Work out the finished part from the listing and answer in its coordinate system (mm). Face numbers are marked on the shaded views. A direction names the side the tool comes from. Coordinates: 2 decimals unless noted, no trailing zeros. Order: outer loops, then holes, each group sorted by start corner. A loop starts at its lowest first (then second) coordinate and runs counter-clockwise, first axis right, second up.
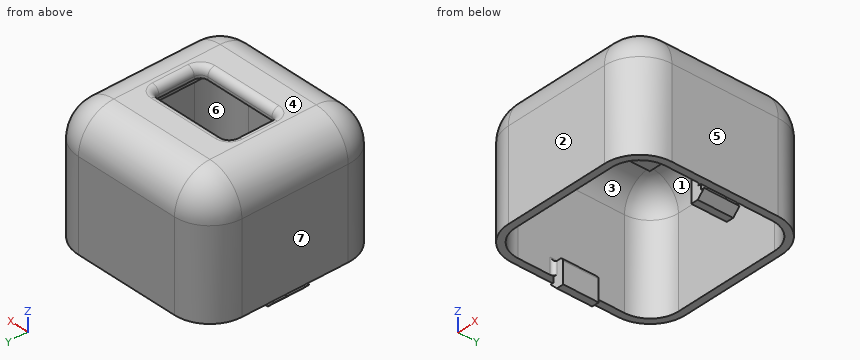
```python
from build123d import *

# Parameters (mm, degrees)
SKETCH1_W                = 50
SKETCH1_H                = 50
BOSS_EXTRUDE1_DEPTH      = 45
FILLET1_R                = 10
SHELL1_T                 = -2
SKETCH2_W                = 24
SKETCH2_H                = 14
CUT_EXTRUDE1_DEPTH       = 10
SKETCH3_W                = 28
SKETCH3_H                = 18
BOSS_EXTRUDE2_DEPTH      = 2
SKETCH4_W                = 24
SKETCH4_H                = 14
CUT_EXTRUDE2_DEPTH       = 2
FILLET2_R                = 2
FILLET3_R                = 2
SKETCH5_W                = 28
SKETCH5_H                = 28
BOSS_EXTRUDE3_DEPTH      = 2
CUT_EXTRUDE4_DEPTH       = 2
SKETCH8_W                = 25
SKETCH8_H                = 17
CUT_EXTRUDE5_DEPTH       = 1.2
SKETCH9_W                = 28
SKETCH9_H                = 4
CUT_EXTRUDE6_DEPTH       = 1.2
CUT_EXTRUDE10_START      = -10
CUT_EXTRUDE10_DEPTH      = 10
SKETCH14_W               = 7
SKETCH14_H               = 10
BOSS_EXTRUDE4_DEPTH      = 3
SKETCH15_W               = 2
SKETCH15_H               = 10
BOSS_EXTRUDE5_DEPTH      = 1
CHAMFER1_SIZE            = 2
FILLET4_R                = 1
CHAMFER1_OF_MIRROR1_SIZE = 2
FILLET5_R                = 1


with BuildPart() as part:
    # Sketch1 → Boss-Extrude1 (new body)
    with BuildSketch(Plane.XY):
        Rectangle(SKETCH1_W, SKETCH1_H)
    extrude(amount=BOSS_EXTRUDE1_DEPTH)

    # Fillet1
    fillet1_edges = [part.edges().sort_by_distance(p)[0] for p in [
        (-25, 0, 45),
        (0, -25, 45),
        (25, 0, 45),
        (25, -25, 22.5),
        (-25, -25, 22.5),
        (-25, 25, 22.5),
        (25, 25, 22.5),
        (0, 25, 45),
    ]]
    fillet(fillet1_edges, radius=FILLET1_R)

    # Shell1
    shell1_openings = [part.faces().sort_by_distance(p)[0] for p in [
        (0, 0, 0),
    ]]
    offset(amount=SHELL1_T, openings=shell1_openings, kind=Kind.INTERSECTION)

    # Sketch2 → Cut-Extrude1 (cut)
    with BuildSketch(Plane(origin=(0, 0, 43), x_dir=(-1, 0, 0), z_dir=(0, 0, -1))):
        Rectangle(SKETCH2_W, SKETCH2_H)
    extrude(amount=-CUT_EXTRUDE1_DEPTH, mode=Mode.SUBTRACT)

    # Sketch3 → Boss-Extrude2 (add)
    with BuildSketch(Plane(origin=(0, 0, 43), x_dir=(-1, 0, 0), z_dir=(0, 0, -1))):
        Rectangle(SKETCH3_W, SKETCH3_H)
    extrude(amount=BOSS_EXTRUDE2_DEPTH)

    # Sketch4 → Cut-Extrude2 (cut)
    with BuildSketch(Plane.XY.offset(43)):
        Rectangle(SKETCH4_W, SKETCH4_H)
    extrude(amount=-CUT_EXTRUDE2_DEPTH, mode=Mode.SUBTRACT)

    # Fillet2
    fillet2_edges = [part.edges().sort_by_distance(p)[0] for p in [
        (-12, 7, 43),
        (-12, -7, 43),
        (12, -7, 43),
        (12, 7, 43),
    ]]
    fillet(fillet2_edges, radius=FILLET2_R)

    # Fillet3
    fillet3_edges = [part.edges().sort_by_distance(p)[0] for p in [
        (12, 0, 45),
        (0, 7, 45),
        (0, -7, 45),
        (-12, 0, 45),
        (11.414213562, 6.414213562, 45),
        (11.414213562, -6.414213562, 45),
        (-11.414213562, -6.414213562, 45),
        (-11.414213562, 6.414213562, 45),
    ]]
    fillet(fillet3_edges, radius=FILLET3_R)

    # Sketch5 → Boss-Extrude3 (add)
    with BuildSketch(Plane(origin=(0, 0, 41), x_dir=(-1, 0, 0), z_dir=(0, 0, -1))):
        Rectangle(SKETCH5_W, SKETCH5_H)
    extrude(amount=-BOSS_EXTRUDE3_DEPTH)

    # Sketch7 → Cut-Extrude4 (cut)
    with BuildSketch(Plane.XY.offset(43)):
        with BuildLine():
            Line((12, -5), (12, 5))
            ThreePointArc((12, 5), (11.414213562, 6.414213562), (10, 7))
            Line((10, 7), (-10, 7))
            ThreePointArc((-10, 7), (-11.414213562, 6.414213562), (-12, 5))
            Line((-12, 5), (-12, -5))
            ThreePointArc((-12, -5), (-11.414213562, -6.414213562), (-10, -7))
            Line((-10, -7), (10, -7))
            ThreePointArc((10, -7), (11.414213562, -6.414213562), (12, -5))
        make_face()
    extrude(amount=-CUT_EXTRUDE4_DEPTH, mode=Mode.SUBTRACT)

    # Sketch8 → Cut-Extrude5 (cut)
    with BuildSketch(Plane(origin=(0, 0, 41), x_dir=(-1, 0, 0), z_dir=(0, 0, -1))):
        Rectangle(SKETCH8_W, SKETCH8_H)
    extrude(amount=-CUT_EXTRUDE5_DEPTH, mode=Mode.SUBTRACT)

    # Sketch9 → Cut-Extrude6 (cut)
    with BuildSketch(Plane(origin=(0, 0, 41), x_dir=(-1, 0, 0), z_dir=(0, 0, -1))):
        with Locations((0, -12)):
            Rectangle(SKETCH9_W, SKETCH9_H)
    extrude(amount=-CUT_EXTRUDE6_DEPTH, mode=Mode.SUBTRACT)

    # Sketch13 → Cut-Extrude10 (cut)
    with BuildSketch(Plane(origin=(0, 0, 0), x_dir=(-1, 0, 0), z_dir=(0, 0, -1)).offset(CUT_EXTRUDE10_START)):
        with BuildLine():
            Line((-15, -25), (15, -25))
            ThreePointArc((15, -25), (22.071067812, -22.071067812), (25, -15))
            Line((25, -15), (25, 15))
            ThreePointArc((25, 15), (22.071067812, 22.071067812), (15, 25))
            Line((15, 25), (-15, 25))
            ThreePointArc((-15, 25), (-22.071067812, 22.071067812), (-25, 15))
            Line((-25, 15), (-25, -15))
            ThreePointArc((-25, -15), (-22.071067812, -22.071067812), (-15, -25))
        make_face()
    extrude(amount=CUT_EXTRUDE10_DEPTH, mode=Mode.SUBTRACT)

    # Sketch14 → Boss-Extrude4 (add)
    with BuildSketch(Plane(origin=(-23, 0, 0), x_dir=(0, 0, -1), z_dir=(1, 0, 0))):
        with Locations((-10, 0)):
            Rectangle(SKETCH14_W, SKETCH14_H)
    boss_extrude4 = extrude(amount=BOSS_EXTRUDE4_DEPTH)

    # Sketch15 → Boss-Extrude5 (add)
    with BuildSketch(Plane.ZY.offset(23)):
        with Locations((7.5, 0)):
            Rectangle(SKETCH15_W, SKETCH15_H)
    boss_extrude5 = extrude(amount=BOSS_EXTRUDE5_DEPTH)

    # Chamfer1
    chamfer1_edges = [part.edges().sort_by_distance(p)[0] for p in [
        (-24, 0, 6.5),
    ]]
    chamfer(chamfer1_edges, length=CHAMFER1_SIZE - 0.0001)  # a hair under: the kernel refuses the full size

    # Fillet4
    fillet4_edges = [part.edges().sort_by_distance(p)[0] for p in [
        (-23, 5, 11.75),
        (-23, 0, 13.5),
        (-23, -5, 11.75),
        (-20, 0, 13.5),
    ]]
    fillet(fillet4_edges, radius=FILLET4_R)

    # Mirror1: Boss-Extrude4, Boss-Extrude5 across plane
    add(boss_extrude4.mirror(Plane(origin=(0, 0, 0), x_dir=(0, 0, 1), z_dir=(1, 0, 0))))
    add(boss_extrude5.mirror(Plane(origin=(0, 0, 0), x_dir=(0, 0, 1), z_dir=(1, 0, 0))))

    # Chamfer1 of Mirror1
    chamfer1_of_mirror1_edges = [part.edges().sort_by_distance(p)[0] for p in [
        (24, 0, 6.5),
    ]]
    chamfer(chamfer1_of_mirror1_edges, length=CHAMFER1_OF_MIRROR1_SIZE - 0.0001)  # a hair under: the kernel refuses the full size

    # Fillet5
    fillet5_edges = [part.edges().sort_by_distance(p)[0] for p in [
        (23, 5, 11.75),
        (23, 0, 13.5),
        (23, -5, 11.75),
        (20, 0, 13.5),
    ]]
    fillet(fillet5_edges, radius=FILLET5_R)


solid = part.part
```
1. The part is cut by section B-B (z = 15.5). Determine the outline of the cut face in (x, y).
2. Consider probe 1 along X at (y, z) = (-11.5, 30); probe 2 along Z at (x, y) = (6, -9). Determine where each line is inside the solid, lowest interval first.
3. The mould has two halves that part along X. Classify the marked faces 4, 5, 6 and 7: released by +X, released by -X, zero draft, split by the parting line, or undercut.
4. For the marked faces 1, 2 and 3, determine the directions among +Z, -Z, +X, -X, +Y, -Y from which every point of the face is accessible in a straight line to the end or side of a thin tool.
5. Flat-ended cylindrical pins translate along their axes: pin 1 (2 mm diameter, centred on x = 22.5, z = 11.5, fed in from +Y); pin 2 (1.2 mm diameter, centred on x = -22.5, z = 11.5, fed in from -Y); pin 3 (4.5 mm diameter, centred on x = -23, z = 9.5, fed in from +Y). Find the tip coordinate at first contact, or state that the pin passes through.
6. The part is cut by section D-D (z = 40). Determine the outline of the cut face in (x, y) (1 decimal), plus the area to 3 significant figures.
7. The part is cut by section C-C (y = 16.5). Determine the outline of the cut face in (x, z), plus the area to 3 significant figures.
8. The part is cut by section A-A (x = 0). Determine the outline of the cut face in (y, z).
Worked out:
1. outline: (-25, -15) arc R10 ccw to (-15, -25) - (15, -25) arc R10 ccw to (25, -15) - (25, 15) arc R10 ccw to (15, 25) - (-15, 25) arc R10 ccw to (-25, 15) - close; hole (-23, -15) arc R8 ccw to (-15, -23) - (15, -23) arc R8 ccw to (23, -15) - (23, 15) arc R8 ccw to (15, 23) - (-15, 23) arc R8 ccw to (-23, 15) - close
2. probe 1: x = -25 to -23, 23 to 25
2. probe 2: z = 41 to 45
3. face 4: zero draft
3. face 5: released by +X
3. face 6: undercut
3. face 7: released by -X
4. face 1: -Z
4. face 2: +Z, -Z, +X, -X, -Y
4. face 3: none
5. pin 1: stops at y = 22.6
5. pin 2: stops at y = -22.24
5. pin 3: stops at y = 23.14
6. outline: (-23.7, -15) arc R8.7 ccw to (-15, -23.7) - (15, -23.7) arc R8.7 ccw to (23.7, -15) - (23.7, 15) arc R8.7 ccw to (15, 23.7) - (-15, 23.7) arc R8.7 ccw to (-23.7, 15) - close; hole (-21.2, -15) arc R6.2 ccw to (-15, -21.2) - (15, -21.2) arc R6.2 ccw to (21.2, -15) - (21.2, 15) arc R6.2 ccw to (15, 21.2) - (-15, 21.2) arc R6.2 ccw to (-21.2, 15) - close
6. area: 403 mm2
7. outline: (-24.89, 10) - (-22.86, 10) - (-22.86, 35) arc R7.86 cw to (-15, 42.86) - (15, 42.86) arc R7.86 cw to (22.86, 35) - (22.86, 10) - (24.89, 10) - (24.89, 35) arc R9.89 ccw to (15, 44.89) - (-15, 44.89) arc R9.89 ccw to (-24.89, 35) - close
7. area: 219 mm2
8. outline: (-25, 10) - (-23, 10) - (-23, 35) arc R8 cw to (-15, 43) - (-14, 43) - (-14, 42.2) - (-10, 42.2) - (-10, 41) - (-8.5, 41) - (-8.5, 42.2) - (-7, 42.2) - (-7, 43) arc R2 ccw to (-9, 45) - (-15, 45) arc R10 ccw to (-25, 35) - close; (7, 42.2) - (8.5, 42.2) - (8.5, 41) - (14, 41) - (14, 43) - (15, 43) arc R8 cw to (23, 35) - (23, 10) - (25, 10) - (25, 35) arc R10 ccw to (15, 45) - (9, 45) arc R2 ccw to (7, 43) - close
